```python
from build123d import *

# Parameters (mm, degrees)
SKETCH1_W           = 45
SKETCH1_H           = 20
BOSS_EXTRUDE1_DEPTH = 1
SKETCH2_R           = 8
BOSS_EXTRUDE2_DEPTH = 12


with BuildPart() as part:
    # Sketch1 → Boss-Extrude1 (new body)
    with BuildSketch(Plane.XY):
        Rectangle(SKETCH1_W, SKETCH1_H)
    extrude(amount=BOSS_EXTRUDE1_DEPTH)

    # Sketch2 → Boss-Extrude2 (add)
    with BuildSketch(Plane.XY.offset(1)):
        with Locations(Location((-12.5, 0, 0), (0, 0, 180))):
            Circle(SKETCH2_R)
    boss_extrude2 = extrude(amount=BOSS_EXTRUDE2_DEPTH)

    # Mirror1: Boss-Extrude2 across plane
    add(boss_extrude2.mirror(Plane(origin=(0, 0, 0), x_dir=(0, 0, 1), z_dir=(1, 0, 0))))


solid = part.part
```
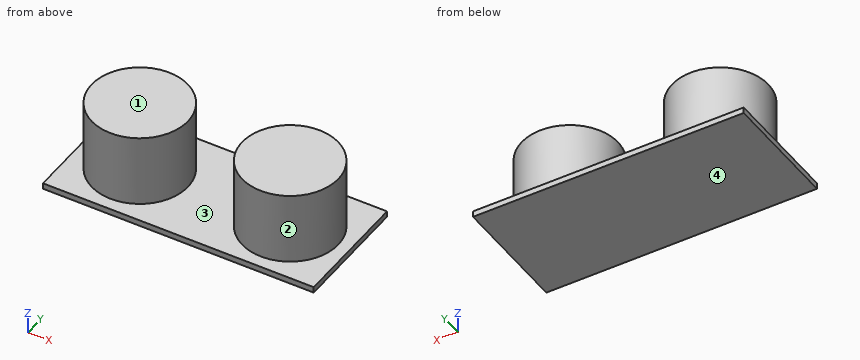
Verification items for the finished model (mm, model axes). Face numbers are marked on the shaded views. A direction names the side the tool comes from. Round coordinates to 2 decimals unless told otherwise and drop trailing zeros. Order: outer loops, then holes, each group sorted by start corner. A loop starts at its lowest first (then second) coordinate and runs counter-clockwise, first axis right, second up. Notation, with made-up numbers: (6.5, 53) -> (45.5, 53) arc R12 cw to (45.5, 65) -> close; hole circle Ø5 at (-11.75, 54). An arc over 180 degrees is marked (long way). Put each result on its own line as item: value. Start each with the question number.
(1) Depth check by flat-ended pin: pin 1 Ø3 at (x, z) = (6.5, 6) entering from -Y; pin 2 Ø6 at (y, z) = (-4.5, 9) entering from -X; pin 3 Ø1 at (y, z) = (-6.5, 9.5) entering from +X. Enter the tip coordinate at first touch or a pass-through.
(2) Section check D-D (y = -3.25). Enter the section's corners in (x, z), then the cut area to 3 significant figures.
(3) Section check B-B (z = 10.75). Enter the section's corners in (x, y).
(4) Section check C-C (y = 0). Enter the section's corners in (x, z).
(5) Tool access check on the marked faces 3 and 4. Record the directions out of +Z, -Z, +X, -X, +Y, -Y that give a thin tool (end or side, any length) a straight path to the whole face; none if there is none.
(6) Material ranges on line 1 along Z through (x, y) = (0.5, 6); line 2 along X through (y, z) = (7.25, 11.75); line 3 along X through (y, z) = (1, 7), recorded low to high.
(7) Draft check along X on the marked faces 1 and 2. Enter one of: +X half, -X half, draft (parallel to the pull), parting line (faces both ways), or undercut.
(8) Section check A-A (x = -12.5). Enter the section's corners in (y, z).
Completed:
1. pin 1: stops at y = -6.61
1. pin 2: stops at x = -20.36
1. pin 3: stops at x = 17.79
2. outline: (-22.5, 0) -> (22.5, 0) -> (22.5, 1) -> (19.81, 1) -> (19.81, 13) -> (5.19, 13) -> (5.19, 1) -> (-5.19, 1) -> (-5.19, 13) -> (-19.81, 13) -> (-19.81, 1) -> (-22.5, 1) -> close
2. area: 396 mm2
3. outline: circle Ø16 at (-12.5, 0); circle Ø16 at (12.5, 0)
4. outline: (-22.5, 0) -> (22.5, 0) -> (22.5, 1) -> (20.5, 1) -> (20.5, 13) -> (4.5, 13) -> (4.5, 1) -> (-4.5, 1) -> (-4.5, 13) -> (-20.5, 13) -> (-20.5, 1) -> (-22.5, 1) -> close
5. face 3: +Z
5. face 4: -Z, +X, -X, +Y, -Y
6. line 1: z = 0 to 1
6. line 2: x = -15.88 to -9.12, 9.12 to 15.88
6. line 3: x = -20.44 to -4.56, 4.56 to 20.44
7. face 1: draft
7. face 2: undercut
8. outline: (-10, 0) -> (10, 0) -> (10, 1) -> (8, 1) -> (8, 13) -> (-8, 13) -> (-8, 1) -> (-10, 1) -> close
